```python
from build123d import *

# Parameters (mm, degrees)
SKETCH_W     = 42
SKETCH_H     = 32
PAD_DEPTH    = 2
POCKET_DEPTH = 2.001
SKETCH004_W  = 1.8
SKETCH004_H  = 32
PAD001_DEPTH = 6
PAD002_DEPTH = 1
PAD003_DEPTH = 1
FILLET_R     = 0.99
FILLET001_R  = 5
FILLET002_R  = 0.3


with BuildPart() as part:
    # Sketch → Pad (new body)
    with BuildSketch(Plane.XY):
        Rectangle(SKETCH_W, SKETCH_H)
    extrude(amount=PAD_DEPTH)

    # Sketch001 (on Face6 of Pad) → Pocket (cut, through all)
    with BuildSketch(Plane.XY.offset(2)):
        with BuildLine():
            Line((-11, 12.5), (11, 12.5))
            ThreePointArc((12.5, 11), (12.06066, 12.06066), (11, 12.5))
            Line((12.5, 11), (12.5, -11))
            ThreePointArc((11, -12.5), (12.06066, -12.06066), (12.5, -11))
            Line((11, -12.5), (-11, -12.5))
            ThreePointArc((-12.5, -11), (-12.06066, -12.06066), (-11, -12.5))
            Line((-12.5, -11), (-12.5, 11))
            ThreePointArc((-11, 12.5), (-12.06066, 12.06066), (-12.5, 11))
        make_face()
    extrude(amount=-POCKET_DEPTH, mode=Mode.SUBTRACT)

    # Sketch004 (on Face5 of Pocket) → Pad001 (join)
    with BuildSketch(Plane.XY.offset(2)):
        with Locations((-20.1, 0)):
            Rectangle(SKETCH004_W, SKETCH004_H)
        with Locations((20.1, 0)):
            Rectangle(SKETCH004_W, SKETCH004_H)
    extrude(amount=PAD001_DEPTH)

    # Sketch005 (on Face22 of Pad001) → Pad002 (join)
    with BuildSketch(Plane.YZ.offset(-19.2)):
        with BuildLine():
            ThreePointArc((-5, 7.5), (-6.5, 6), (-5, 4.5))
            Line((-5, 4.5), (5, 4.5))
            ThreePointArc((5, 4.5), (6.5, 6), (5, 7.5))
            Line((-5, 7.5), (5, 7.5))
        make_face()
    extrude(amount=PAD002_DEPTH)

    # Sketch006 (on Face23 of Pad002) → Pad003 (join)
    with BuildSketch(Plane(origin=(19.2, 0, 0), x_dir=(0, -1, 0), z_dir=(-1, 0, 0))):
        with BuildLine():
            ThreePointArc((-5, 7.5), (-6.5, 6), (-5, 4.5))
            Line((-5, 4.5), (5, 4.5))
            ThreePointArc((5, 4.5), (6.5, 6), (5, 7.5))
            Line((-5, 7.5), (5, 7.5))
        make_face()
    extrude(amount=PAD003_DEPTH)

    # Fillet
    fillet_edges = [part.edges().sort_by_distance(p)[0] for p in [
        (18.2, 6.5, 6),
        (18.2, 0, 4.5),
        (18.2, -6.5, 6),
        (18.2, 0, 7.5),
        (-18.2, -6.5, 6),
        (-18.2, 0, 4.5),
        (-18.2, 6.5, 6),
        (-18.2, 0, 7.5),
    ]]
    fillet(fillet_edges, radius=FILLET_R)

    # Fillet001
    fillet001_edges = [part.edges().sort_by_distance(p)[0] for p in [
        (20.1, 16, 8),
        (20.1, -16, 8),
        (-20.1, 16, 8),
        (-20.1, -16, 8),
    ]]
    fillet(fillet001_edges, radius=FILLET001_R)

    # Fillet002
    fillet002_edges = [part.edges().sort_by_distance(p)[0] for p in [
        (0, 16, 0),
        (-21, 0, 0),
        (21, 0, 0),
        (0, -16, 0),
        (12.06066, -12.06066, 0),
        (12.5, 0, 0),
        (12.06066, 12.06066, 0),
        (0, 12.5, 0),
        (-12.06066, 12.06066, 0),
        (-12.5, 0, 0),
        (-12.06066, -12.06066, 0),
        (0, -12.5, 0),
    ]]
    fillet(fillet002_edges, radius=FILLET002_R)


solid = part.part
```
Here's how the part is built. I have some questions about the finished solid (model axes, mm). A direction names the side the tool comes from. Give positions to 0.01 mm unless a question says otherwise; leave off trailing zeros. Write each loop counter-clockwise with the first axis right and the second up, starting at its lowest first coordinate (ties: lowest second). Pieces come first, ordered by that corner, then holes. Notation, with made-up numbers: (53, 59.25) -> (110, 59.25) arc R19 cw to (110, 90.25) -> close; hole circle Ø2 at (-7, 30). An arc over 180 degrees is marked (long way). Use one line per item in the form item = value.
1) I'm going to push a flat-ended pin straight in: pin 1 (1 mm diameter, centred on x = 13, y = -8, fed in from +Z). Where does the tip first touch, or does it pass through?
Verdict:
pin_1 = 2
2) Suppose I cut it at C-C (x = -15). Please give me the cut outline in (y, z).
Verdict:
outline = (-16, 0.3) arc R0.3 ccw to (-15.7, 0) -> (15.7, 0) arc R0.3 ccw to (16, 0.3) -> (16, 2) -> (-16, 2) -> close
3) We'd pull the mould along Z, two halves only. Please class faces 5 (the face through (-12.05, 12.07, 1.16)), 6 (the face through (-20, 14, 7)), 7 (the face through (18.5, -0.07, 4.78)): +Z half, -Z half, draft (parallel to the pull), parting line (faces both ways), or undercut.
Verdict:
face_5 = draft
face_6 = +Z half
face_7 = undercut
4) If I drill on L1, parallel to X at y = 8.5, z = 7.25; L2, parallel to X at y = -2.5, z = 5.5; L3, parallel to Y at x = 9.5, z = 1, over which ranges is the centre line in solid material (lowest first)? Write a range as [from, to].
Verdict:
L1 = [-21, -19.2], [19.2, 21]
L2 = [-21, -18.2], [18.2, 21]
L3 = [-16, -12.5], [12.5, 16]
5) On a 3-axis mill with a long thin cutter (end or side, diameter ignored), from which of +Z, -Z, +X, -X, +Y, -Y can I reach the whole of each face in a straight line? I mean faces 1 (the face through (12.05, -12.07, 1.16)), 2 (the face through (0, -16, 1)), 3 (the face through (19.2, 0, 4)), 4 (the face through (-18.2, 0, 6)). Say none if no direction works.
Verdict:
face_1 = +Z, -Z
face_2 = +Z, -Z, +X, -X, -Y
face_3 = none
face_4 = +Z, +Y, -Y
6) Suppose I cut it at A-A (x = 3.5). Please give me the cut outline in (y, z), and give its area (3 significant figures).
Verdict:
outline = (-16, 0.3) arc R0.3 ccw to (-15.7, 0) -> (-12.8, 0) arc R0.3 ccw to (-12.5, 0.3) -> (-12.5, 2) -> (-16, 2) -> close; (12.5, 0.3) arc R0.3 ccw to (12.8, 0) -> (15.7, 0) arc R0.3 ccw to (16, 0.3) -> (16, 2) -> (12.5, 2) -> close
area = 13.9 mm2
